```python
from build123d import *

# Parameters (mm, degrees)
SKETCH1_W           = 70
SKETCH1_H           = 70
SKETCH1_R           = 23.5
SKETCH1_R_2         = 1
SKETCH1_R_3         = 1.5
BOSS_EXTRUDE1_DEPTH = 7


with BuildPart() as part:
    # Sketch1 → Boss-Extrude1 (new body)
    with BuildSketch(Plane(origin=(0, 0, 0), x_dir=(1, 0, 0), z_dir=(0, 1, 0))):
        Rectangle(SKETCH1_W, SKETCH1_H)
        with Locations(Location((0, 0, 0), (0, 0, 270))):
            Circle(SKETCH1_R, mode=Mode.SUBTRACT)
        with Locations(Location((0, 27.5, 0), (0, 0, 270))):
            Circle(SKETCH1_R_2, mode=Mode.SUBTRACT)
        with Locations(Location((23.815698604, 13.75, 0), (0, 0, 270))):
            Circle(SKETCH1_R_2, mode=Mode.SUBTRACT)
        with Locations(Location((23.815698604, -13.75, 0), (0, 0, 270))):
            Circle(SKETCH1_R_2, mode=Mode.SUBTRACT)
        with Locations(Location((0, -27.5, 0), (0, 0, 270))):
            Circle(SKETCH1_R_2, mode=Mode.SUBTRACT)
        with Locations(Location((-23.815698604, -13.75, 0), (0, 0, 270))):
            Circle(SKETCH1_R_2, mode=Mode.SUBTRACT)
        with Locations(Location((-23.815698604, 13.75, 0), (0, 0, 270))):
            Circle(SKETCH1_R_2, mode=Mode.SUBTRACT)
        with Locations(Location((-31.392589354, -8.411618966, 0), (0, 0, 270))):
            Circle(SKETCH1_R_3, mode=Mode.SUBTRACT)
        with Locations(Location((-31.392589354, 8.411618966, 0), (0, 0, 270))):
            Circle(SKETCH1_R_3, mode=Mode.SUBTRACT)
        with Locations(Location((-22.980970389, 22.980970389, 0), (0, 0, 270))):
            Circle(SKETCH1_R_3, mode=Mode.SUBTRACT)
        with Locations(Location((-8.411618966, 31.392589354, 0), (0, 0, 270))):
            Circle(SKETCH1_R_3, mode=Mode.SUBTRACT)
        with Locations(Location((8.411618966, 31.392589354, 0), (0, 0, 270))):
            Circle(SKETCH1_R_3, mode=Mode.SUBTRACT)
        with Locations(Location((22.980970389, 22.980970389, 0), (0, 0, 270))):
            Circle(SKETCH1_R_3, mode=Mode.SUBTRACT)
        with Locations(Location((31.392589354, 8.411618966, 0), (0, 0, 270))):
            Circle(SKETCH1_R_3, mode=Mode.SUBTRACT)
        with Locations(Location((31.392589354, -8.411618966, 0), (0, 0, 270))):
            Circle(SKETCH1_R_3, mode=Mode.SUBTRACT)
        with Locations(Location((22.980970389, -22.980970389, 0), (0, 0, 270))):
            Circle(SKETCH1_R_3, mode=Mode.SUBTRACT)
        with Locations(Location((8.411618966, -31.392589354, 0), (0, 0, 270))):
            Circle(SKETCH1_R_3, mode=Mode.SUBTRACT)
        with Locations(Location((-8.411618966, -31.392589354, 0), (0, 0, 270))):
            Circle(SKETCH1_R_3, mode=Mode.SUBTRACT)
        with Locations(Location((-22.980970389, -22.980970389, 0), (0, 0, 270))):
            Circle(SKETCH1_R_3, mode=Mode.SUBTRACT)
    extrude(amount=BOSS_EXTRUDE1_DEPTH)


solid = part.part
```
Work out the finished part from the listing and answer in its coordinate system (mm). Coordinates: 2 decimals unless noted, no trailing zeros. Loops run counter-clockwise (first coordinate to the right, second up) from the corner with the lowest first, then second, coordinate; pieces in that order, holes last. Notation, with made-up numbers: (86, 26) -> (103, 26) arc R19 cw to (103, 51) -> close; hole circle Ø10 at (79.25, 60.25). An arc over 180 degrees is marked (long way). Answer as CSV lines item,"result".
Q1. The part is cut by section A-A on z = -27.5. Write down the section's boundary in (x, y).
Findings:
outline,"(-35, 0) -> (-1, 0) -> (-1, 7) -> (-35, 7) -> close; (1, 0) -> (35, 0) -> (35, 7) -> (1, 7) -> close"
Q2. The part is cut by section C-C on y = 2.75. State how many separate pieces and enclosed holes the cut face has, and give its area (3 significant figures).
Findings:
separate pieces,"1"
enclosed holes,"19"
area,"3,060 mm²"
Q3. The part is cut by section B-B on x = 4.5. Write down the section's boundary in (y, z), and give its area (3 significant figures).
Findings:
outline,"(0, -35) -> (7, -35) -> (7, -23.07) -> (0, -23.07) -> close; (0, 23.07) -> (7, 23.07) -> (7, 35) -> (0, 35) -> close"
area,"167 mm²"
Q4. The part is cut by section D-D on z = 13.75. Write down the section's boundary in (x, y), and give its area (3 significant figures).
Findings:
outline,"(-35, 0) -> (-24.82, 0) -> (-24.82, 7) -> (-35, 7) -> close; (-22.82, 0) -> (-19.06, 0) -> (-19.06, 7) -> (-22.82, 7) -> close; (19.06, 0) -> (22.82, 0) -> (22.82, 7) -> (19.06, 7) -> close; (24.82, 0) -> (35, 0) -> (35, 7) -> (24.82, 7) -> close"
area,"195 mm²"
Q5. Each of these flat-tipped pins is pushed along its axis until it touches: pin 1 (1.2 mm diameter, centred on x = 23.82, z = 13.75, fed in from -Y); pin 2 (12 mm diameter, centred on x = 3, z = -19, fed in from +Y). Where does it stop, or does it pass through?
Findings:
pin 1,"passes through"
pin 2,"stops at y = 7"
Q6. For a pull along X with two mould halves and no side action, classify faces 1 (the face through (24.659, 3.451, -13.212)), 2 (the face through (-24, 7, 0)), 3 (the face through (35, 3, 0)), 4 (the face through (-8.346, 3.451, 29.894)) as +X half, -X half, draft (parallel to the pull), parting line (faces both ways), or undercut.
Findings:
face 1,"undercut"
face 2,"draft"
face 3,"+X half"
face 4,"undercut"
Q7. Find the intervals of material crossed by probe 1 along X at (y, z) = (2.5, 0); probe 2 along X at (y, z) = (2, 32); probe 3 along Z at (x, y) = (-31.5, 6), in increasing order.
Findings:
probe 1,"x = -35 to -23.5, 23.5 to 35"
probe 2,"x = -35 to -9.78, -7.04 to 7.04, 9.78 to 35"
probe 3,"z = -35 to -9.91, -6.92 to 6.92, 9.91 to 35"
